For this review, take the finished solid that the model builds, in its own axes (mm). A direction names the side the tool comes from. Coordinates: 2 decimals unless noted, no trailing zeros. Loops run counter-clockwise (first coordinate to the right, second up) from the corner with the lowest first, then second, coordinate; pieces in that order, holes last. Notation, with made-up numbers: (39, 32.25) - (66, 32.25) arc R25 cw to (66, 54.25) - close; hole circle Ø1 at (-12, -30.5). An arc over 180 degrees is marked (long way). Use one line per item in the form item = value. Start each with the question number.
1. Draft analysis for pull direction Y (two halves, no side actions). For faces 4 (the face through (-62.4, 0.4, -0.31)), 5 (the face through (-59.2, 3.14, -5.52)), 6 (the face through (-73.025, -3.5, 0.1)), state which applies: +Y half, -Y half, draft (parallel to the pull), parting line (faces both ways), or undercut.
2. Add section A-A on x = 37. Give the boundary of the cut face in (y, z) (3 decimals), and give its area (3 significant figures).
3. Machinability: for faces 1 (the face through (-52.26, -5, -2)), 2 (the face through (-59.2, -3.14, 5.52)), 3 (the face through (-68.526, -3.856, -5.029)), which of the approach directions +Z, -Z, +X, -X, +Y, -Y give a long, thin tool a straight path to every point of the face, cutting with its end or side? Answer none if there is none.
4. For pin 1 Ø3 at (x, y) = (-2, 4.5) entering from +Z; pin 2 Ø3 at (x, z) = (1, 3.5) entering from -Y; pin 3 Ø5.5 at (y, z) = (0, 0) entering from -X; pin 4 Ø2 at (y, z) = (-4, 5.5) entering from -X, all flat-tipped, find the tip position at first contact; note any pin that passes through.
5. To check wall thickness, follow probe 1 along X at (y, z) = (5.5, -3.5) (1 decimal); probe 2 along X at (y, z) = (5.25, 0.25) (1 decimal); probe 3 along Z at (x, y) = (-52, -3.25). State the ranges of each line that lie inside material, in increasing order.
```python
from build123d import *

# Parameters (mm, degrees)
BOSS_EXTRUDE1_DEPTH = 73.025
CUT_EXTRUDE1_START  = -7.8867
SKETCH2_R           = 6.3373
CUT_EXTRUDE1_DEPTH  = 7.8867
CUT_EXTRUDE2_START  = -1.1684
SKETCH3_R           = 5.0292
CUT_EXTRUDE2_DEPTH  = 1.1684
SKETCH4_R           = 3.175
CUT_EXTRUDE3_DEPTH  = 9.02462
CHAMFER1_SIZE       = 1.016


with BuildPart() as part:
    # Sketch1 → Boss-Extrude1 (new, symmetric)
    with BuildSketch(Plane(origin=(0, 0, 0), x_dir=(0, 0, -1), z_dir=(1, 0, 0))):
        with BuildLine():
            Line((2.634981025, 6.35), (-2.634981025, 6.35))
            ThreePointArc((-2.634981025, 6.35), (-3.4375, 5.953924651), (-4.181770802, 5.456960506))
            Line((-4.181770802, 5.456960506), (-6.816751826, 0.893039494))
            ThreePointArc((-6.816751826, 0.893039494), (-6.875, 0), (-6.816751826, -0.893039494))
            Line((-6.816751826, -0.893039494), (-4.181770802, -5.456960506))
            ThreePointArc((-4.181770802, -5.456960506), (-3.4375, -5.953924651), (-2.634981025, -6.35))
            Line((-2.634981025, -6.35), (2.634981025, -6.35))
            ThreePointArc((2.634981025, -6.35), (3.4375, -5.953924651), (4.181770802, -5.456960506))
            Line((4.181770802, -5.456960506), (6.816751826, -0.893039494))
            ThreePointArc((6.816751826, -0.893039494), (6.875, 0), (6.816751826, 0.893039494))
            Line((6.816751826, 0.893039494), (4.181770802, 5.456960506))
            ThreePointArc((4.181770802, 5.456960506), (3.4375, 5.953924651), (2.634981025, 6.35))
        make_face()
    extrude(amount=BOSS_EXTRUDE1_DEPTH, both=True)

    # Sketch2 → Cut-Extrude1 (cut)
    with BuildSketch(Plane.ZY.offset(73.025).offset(CUT_EXTRUDE1_START)):
        with BuildLine():
            Line((-4.181770802, 5.456960506), (-6.816751826, 0.893039494))
            ThreePointArc((-6.816751826, 0.893039494), (-6.875, 0), (-6.816751826, -0.893039494))
            Line((-6.816751826, -0.893039494), (-4.181770802, -5.456960506))
            ThreePointArc((-4.181770802, -5.456960506), (-3.4375, -5.953924651), (-2.634981025, -6.35))
            Line((-2.634981025, -6.35), (2.634981025, -6.35))
            ThreePointArc((2.634981025, -6.35), (3.4375, -5.953924651), (4.181770802, -5.456960506))
            Line((4.181770802, -5.456960506), (6.816751826, -0.893039494))
            ThreePointArc((6.816751826, -0.893039494), (6.875, 0), (6.816751826, 0.893039494))
            Line((6.816751826, 0.893039494), (4.181770802, 5.456960506))
            ThreePointArc((4.181770802, 5.456960506), (3.4375, 5.953924651), (2.634981025, 6.35))
            Line((2.634981025, 6.35), (-2.634981025, 6.35))
            ThreePointArc((-2.634981025, 6.35), (-3.4375, 5.953924651), (-4.181770802, 5.456960506))
        make_face()
        Circle(SKETCH2_R, mode=Mode.SUBTRACT)
    extrude(amount=CUT_EXTRUDE1_DEPTH, mode=Mode.SUBTRACT)

    # Sketch3 → Cut-Extrude2 (cut)
    with BuildSketch(Plane.ZY.offset(53.4289).offset(CUT_EXTRUDE2_START)):
        with BuildLine():
            Line((-4.181770802, 5.456960506), (-6.816751826, 0.893039494))
            ThreePointArc((-6.816751826, 0.893039494), (-6.875, 0), (-6.816751826, -0.893039494))
            Line((-6.816751826, -0.893039494), (-4.181770802, -5.456960506))
            ThreePointArc((-4.181770802, -5.456960506), (-3.4375, -5.953924651), (-2.634981025, -6.35))
            Line((-2.634981025, -6.35), (2.634981025, -6.35))
            ThreePointArc((2.634981025, -6.35), (3.4375, -5.953924651), (4.181770802, -5.456960506))
            Line((4.181770802, -5.456960506), (6.816751826, -0.893039494))
            ThreePointArc((6.816751826, -0.893039494), (6.875, 0), (6.816751826, 0.893039494))
            Line((6.816751826, 0.893039494), (4.181770802, 5.456960506))
            ThreePointArc((4.181770802, 5.456960506), (3.4375, 5.953924651), (2.634981025, 6.35))
            Line((2.634981025, 6.35), (-2.634981025, 6.35))
            ThreePointArc((-2.634981025, 6.35), (-3.4375, 5.953924651), (-4.181770802, 5.456960506))
        make_face()
        Circle(SKETCH3_R, mode=Mode.SUBTRACT)
    extrude(amount=CUT_EXTRUDE2_DEPTH, mode=Mode.SUBTRACT)

    # Sketch4 → Cut-Extrude3 (cut)
    with BuildSketch(Plane.ZY.offset(73.025)):
        Circle(SKETCH4_R)
    extrude(amount=-CUT_EXTRUDE3_DEPTH, mode=Mode.SUBTRACT)

    # Sketch6 → Cut-Revolve1 (revolve, cut)
    with BuildSketch(Plane.XY, mode=Mode.PRIVATE) as cut_revolve1_sk:
        Polygon((-62.09538, 0), (-64.00038, 0), (-64.00038, 3.175), align=None)
    revolve(cut_revolve1_sk.sketch.rotate(Axis((-62.09538, 0, 0), (-1, 0, 0)), 180), axis=Axis((-62.09538, 0, 0), (-1, 0, 0)), mode=Mode.SUBTRACT)

    # Chamfer1
    chamfer1_edges = [part.edges().sort_by_distance(p)[0] for p in [
        (-73.025, 0, -6.3373),
    ]]
    chamfer(chamfer1_edges, length=CHAMFER1_SIZE)


solid = part.part
```
Conclusion:
q1.face_4 = undercut
q1.face_5 = +Y half
q1.face_6 = draft
q2.outline = (-6.35, -2.635) arc R6.875 ccw to (-5.457, -4.182) - (-0.893, -6.817) arc R6.875 ccw to (0.893, -6.817) - (5.457, -4.182) arc R6.875 ccw to (6.35, -2.635) - (6.35, 2.635) arc R6.875 ccw to (5.457, 4.182) - (0.893, 6.817) arc R6.875 ccw to (-0.893, 6.817) - (-5.457, 4.182) arc R6.875 ccw to (-6.35, 2.635) - close
q2.area = 137 mm^2
q3.face_1 = none
q3.face_2 = +Z, +X, -X, -Y
q3.face_3 = -X
q4.pin_1 = 5.6
q4.pin_2 = -6.35
q4.pin_3 = -63.75
q4.pin_4 = -72.55
q5.probe_1 = -65.1 to -53.4, -52.3 to 73
q5.probe_2 = -73 to -53.4, -52.3 to 73
q5.probe_3 = -5.46 to 5.46
